Here's how the part is built. I have some questions about the finished solid (model axes, mm). A direction names the side the tool comes from. Give positions to 0.01 mm unless a question says otherwise; leave off trailing zeros. Loops run counter-clockwise (first coordinate to the right, second up) from the corner with the lowest first, then second, coordinate; pieces in that order, holes last. Notation, with made-up numbers: (-4.5, 43) -> (28.5, 43) arc R15 cw to (28.5, 49) -> close; hole circle Ø5 at (17.5, -25.75). An arc over 180 degrees is marked (long way). Answer in a Markdown table with one row per item. Add a question column.
Item 1: Which directions (+Z, -Z, +X, -X, +Y, -Y) give clear straight access to the entire face, cutting with the end or side of a thin tool? Please do faces 1 (the face through (0, 6, 5)), 2 (the face through (-10, -1, 5)), 3 (the face through (6, 0, 5)), 4 (the face through (0, -6, 5)), 5 (the face through (-6, 0, 5)).
Item 2: If we section it at C-C (x = -0.5): Write out the boundary of the cut face in (y, z).
Item 3: If we section it at B-B (y = 6.75): Write out the boundary of the cut face in (x, z), then the cut area to 3 significant figures.
Item 4: If I drill on line 1 (Y direction, x = -4.25, z = 7.5); line 2 (Y direction, x = 6.5, z = 7.5), over which ranges is the centre line in solid material (lowest first)?
Item 5: For P1, Ø1.5, axis at y = -1, z = 7, coming from the +X side; P2, Ø1.5, axis at x = -5, z = 7, coming from the +Y side; P3, Ø3, axis at x = 5, y = -5, coming from the -Z side; P4, Ø4, axis at y = -6, z = 3.5, coming from the -X side, each with a flat end and sliding along its axis, tell me the tip position at first contact or that it passes through.
Item 6: If we section it at A-A (z = 6): Write out the boundary of the cut face in (x, y) (3 decimals), then the cut area to 3 significant figures.
```python
from build123d import *

# Parameters (mm, degrees)
SKETCH_W             = 20
SKETCH_H             = 20
PAD_DEPTH            = 10
SKETCH001_W          = 15
SKETCH001_H          = 15
POCKET_DEPTH         = 10.001
SKETCH002_R          = 0.025
POCKET001_DEPTH      = 0.001
POCKET001_DEPTH_BACK = 10.001


with BuildPart() as part:
    # Sketch → Pad (new body)
    with BuildSketch(Plane.XY):
        Rectangle(SKETCH_W, SKETCH_H)
    extrude(amount=PAD_DEPTH)

    # Sketch001 → Pocket (cut, through all)
    with BuildSketch(Plane.XY):
        with Locations((7.5, 9.5)):
            Rectangle(SKETCH001_W, SKETCH001_H)
        with Locations((-9.5, 7.5)):
            Rectangle(SKETCH001_W, SKETCH001_H)
        with Locations((9.5, -7.5)):
            Rectangle(SKETCH001_W, SKETCH001_H)
        with Locations((-7.5, -9.5)):
            Rectangle(SKETCH001_W, SKETCH001_H)
    extrude(amount=POCKET_DEPTH, mode=Mode.SUBTRACT)

    # Sketch002 → Pocket001 (cut, two sides)
    with BuildSketch(Plane.XY) as pocket001_sk:
        Circle(SKETCH002_R)
    extrude(amount=-POCKET001_DEPTH, mode=Mode.SUBTRACT)
    extrude(pocket001_sk.sketch, amount=POCKET001_DEPTH_BACK, mode=Mode.SUBTRACT)


solid = part.part
```
Recorded:
| question | item | result |
|---|---|---|
| 1 | face 1 | +Z, -Z, +X, +Y |
| 1 | face 2 | +Z, -Z, -X, +Y, -Y |
| 1 | face 3 | +Z, -Z, +X, -Y |
| 1 | face 4 | +Z, -Z, -X, -Y |
| 1 | face 5 | +Z, -Z, -X, +Y |
| 2 | outline | (-2, 0) -> (10, 0) -> (10, 10) -> (-2, 10) -> close |
| 3 | outline | (-2, 0) -> (0, 0) -> (0, 10) -> (-2, 10) -> close |
| 3 | area | 20.0 mm^2 |
| 4 | line 1 | y = -2 to 0 |
| 4 | line 2 | y = 0 to 2 |
| 5 | P1 | stops at x = 2 |
| 5 | P2 | stops at y = 0 |
| 5 | P3 | passes through |
| 5 | P4 | stops at x = 0 |
| 6 | outline | (-10, -2) -> (0, -2) -> (0, -10) -> (2, -10) -> (2, 0) -> (10, 0) -> (10, 2) -> (0, 2) -> (0, 10) -> (-2, 10) -> (-2, 0) -> (-10, 0) -> close; hole circle Ø0.05 at (0, 0) |
| 6 | area | 80.0 mm^2 |
